from build123d import *

# Parameters (mm, degrees)
SKETCH_1_R          = 26
SKETCH_1_R_2        = 20
EXTRUDE_1_DEPTH     = 7
SKETCH_2_R          = 25
SKETCH_2_R_2        = 21.5
CUT_EXTRUDE_1_DEPTH = 0.5
SKETCH_3_R          = 24.5
SKETCH_3_R_2        = 23.5
CUT_EXTRUDE_2_DEPTH = 0.8
CUT_EXTRUDE_2_DRAFT = -17


with BuildPart() as part:
    # Эскиз1 → Бобышка-Вытянуть1 (new body)
    with BuildSketch(Plane(origin=(0, 0, 0), x_dir=(1, 0, 0), z_dir=(0, 1, 0))):
        with Locations(Location((0, 0, 0), (0, 0, 270))):
            Circle(SKETCH_1_R)
        with Locations(Location((0, 0, 0), (0, 0, 270))):
            Circle(SKETCH_1_R_2, mode=Mode.SUBTRACT)
    extrude(amount=EXTRUDE_1_DEPTH)

    # Эскиз2 → Вырез-Вытянуть1 (cut)
    with BuildSketch(Plane(origin=(0, 7, 0), x_dir=(1, 0, 0), z_dir=(0, 1, 0))):
        with Locations(Location((0, 0, 0), (0, 0, 270))):
            Circle(SKETCH_2_R)
        with Locations(Location((0, 0, 0), (0, 0, 270))):
            Circle(SKETCH_2_R_2, mode=Mode.SUBTRACT)
    extrude(amount=-CUT_EXTRUDE_1_DEPTH, mode=Mode.SUBTRACT)


with BuildPart() as cut_extrude_2_tool:
    # Эскиз3 → Вырез-Вытянуть2 (with draft: the straight prism first)
    with BuildSketch(Plane(origin=(0, 6.5, 0), x_dir=(1, 0, 0), z_dir=(0, 1, 0))):
        Circle(SKETCH_3_R)
        Circle(SKETCH_3_R_2, mode=Mode.SUBTRACT)
    extrude(amount=-CUT_EXTRUDE_2_DEPTH)
    # Вырез-Вытянуть2: the draft: its side faces are tilted about the plane it starts from
    cut_extrude_2_sides = [cut_extrude_2_tool.faces().sort_by_distance(p)[0] for p in [
        (-24.5, 6.1, 0),
        (-23.5, 6.1, 0),
    ]]
    draft(cut_extrude_2_sides, Plane(origin=(0, 6.5, 0), x_dir=(1, 0, 0), z_dir=(0, 1, 0)), CUT_EXTRUDE_2_DRAFT)


with BuildPart() as part_1:
    add(part.part)

    # Вырез-Вытянуть2: cut by cut_extrude_2_tool
    add(cut_extrude_2_tool.part, mode=Mode.SUBTRACT)


solid = part_1.part
Can you work these out from the model? Positions are in its coordinate system, mm. A direction names the side the tool comes from. Coordinates: 2 decimals unless noted, no trailing zeros. Loops run counter-clockwise (first coordinate to the right, second up) from the corner with the lowest first, then second, coordinate; pieces in that order, holes last. Notation, with made-up numbers: (-17, 70) - (17, 70) arc R19 cw to (17, 91) - close; hole circle Ø3 at (19.25, 81.5). An arc over 180 degrees is marked (long way). Put each result on its own line as item: value. Start each with the question number.
Item 1: Suppose I cut it at A-A (z = 0). Please give me the cut outline in (x, y).
Item 2: Suppose I cut it at C-C (y = 2.25). Please give me the cut outline in (x, z), and give its area (3 significant figures).
Item 3: If we mould it in two halves opening along Z, with no side actions, what happens to faces 1 (the face through (-15.821, 3.451, -20.633)), 2 (the face through (-15.3, 0, 13.4)), 3 (the face through (14.531, 6.754, -15.846))? For each: +Z half, -Z half, draft (parallel to the pull), parting line (faces both ways), or undercut.
Item 4: For pin 1 (2 mm diameter, centred on y = 5.5, z = 18.5, fed in from -X); pin 2 (1 mm diameter, centred on x = -12, y = 1, fed in from +Z); pin 3 (2 mm diameter, centred on x = -12, y = 5, fed in from -Z), each with a flat end and sliding along its axis, tell me the tip position at first contact or that it passes through.
Item 5: If I drill on line 1 along X through (y, z) = (1.5, 0); line 2 along X through (y, z) = (6, -5); line 3 along Z through (x, y) = (-18, 6.25), over which ranges is the centre line in solid material (lowest first)?
Item 6: Which directions (+Z, -Z, +X, -X, +Y, -Y) give clear straight access to the entire face, cutting with the end or side of a thin tool? Please do faces 4 (the face through (-13, 7, 16)), 5 (the face through (7.509, 6.754, 23.846)).
Item 7: Suppose I cut it at B-B (x = 0). Please give me the cut outline in (y, z).
Here are the results:
1. outline: (-26, 0) - (-20, 0) - (-20, 7) - (-21.5, 7) - (-21.5, 6.5) - (-23.5, 6.5) - (-23.74, 5.7) - (-24.26, 5.7) - (-24.5, 6.5) - (-25, 6.5) - (-25, 7) - (-26, 7) - close; (20, 0) - (26, 0) - (26, 7) - (25, 7) - (25, 6.5) - (24.5, 6.5) - (24.26, 5.7) - (23.74, 5.7) - (23.5, 6.5) - (21.5, 6.5) - (21.5, 7) - (20, 7) - close
2. outline: circle Ø52 at (0, 0); hole circle Ø40 at (0, 0)
2. area: 867 mm²
3. face 1: parting line
3. face 2: draft
3. face 3: undercut
4. pin 1: x = -19.23
4. pin 2: z = 23.32
4. pin 3: z = -23.56
5. line 1: -26 to -20, 20 to 26
5. line 2: -25.51 to -23.83, -23.12 to -19.36, 19.36 to 23.12, 23.83 to 25.51
5. line 3: -18.76 to -16.51, -15.23 to -8.72, 8.72 to 15.23, 16.51 to 18.76
6. face 4: +Z, -Z, +X, -X, +Y
6. face 5: +Y
7. outline: (0, -26) - (7, -26) - (7, -25) - (6.5, -25) - (6.5, -24.5) - (5.7, -24.26) - (5.7, -23.74) - (6.5, -23.5) - (6.5, -21.5) - (7, -21.5) - (7, -20) - (0, -20) - close; (0, 20) - (7, 20) - (7, 21.5) - (6.5, 21.5) - (6.5, 23.5) - (5.7, 23.74) - (5.7, 24.26) - (6.5, 24.5) - (6.5, 25) - (7, 25) - (7, 26) - (0, 26) - close
